Read the model definition and answer for the solid it produces. Units are mm, in the model's axes. A direction names the side the tool comes from. Give positions to 0.01 mm unless a question says otherwise; leave off trailing zeros. Order: outer loops, then holes, each group sorted by start corner. A loop starts at its lowest first (then second) coordinate and runs counter-clockwise, first axis right, second up. Notation, with made-up numbers: (39.25, 76.25) - (48.25, 76.25) arc R30 cw to (48.25, 106.25) - close; hole circle Ø3 at (67.25, -0.5). An arc over 180 degrees is marked (long way). Write item = value, one per line.
```python
from build123d import *

# Parameters (mm, degrees)
BOSS_EXTRU_1_DEPTH      = 4
ESQUISSE4_R             = 2.43
ENL_V_MAT_EXTRU_1_DEPTH = 2.7
ESQUISSE5_R             = 0.75
ENL_V_MAT_EXTRU_2_DEPTH = 1.3
CONG_1_R                = 1
ESQUISSE6_W             = 5.35
ESQUISSE6_H             = 23
BOSS_EXTRU_2_DEPTH      = 4
CONG_4_R                = 5.45
ENL_V_START             = -4
ENL_V_MAT_EXTRU_3_DEPTH = 4
CONG_5_R                = 2
CONG_6_R                = 2
CONG_7_R                = 1


with BuildPart() as part:
    # Esquisse3 → Boss.-Extru.1 (new body)
    with BuildSketch(Plane.XY):
        with BuildLine():
            Line((0, 0), (0, 65))
            Line((0, 65), (11.3, 65))
            Line((11.3, 65), (11.3, 11.3))
            Line((11.3, 11.3), (22.73, 11.3))
            Line((22.73, 11.3), (22.73, -23))
            ThreePointArc((22.73, -23), (17.08, -28.65), (11.43, -23))
            Line((11.43, -23), (11.43, 0))
            Line((11.43, 0), (0, 0))
        make_face()
    extrude(amount=BOSS_EXTRU_1_DEPTH)

    # Esquisse4 → Enlèv. mat.-Extru.1 (cut)
    with BuildSketch(Plane.XY.offset(4)):
        with Locations((17.08, -23)):
            Circle(ESQUISSE4_R)
    extrude(amount=-ENL_V_MAT_EXTRU_1_DEPTH, mode=Mode.SUBTRACT)

    # Esquisse5 → Enlèv. mat.-Extru.2 (cut)
    with BuildSketch(Plane.XY.offset(1.3)):
        with Locations((17.08, -23)):
            Circle(ESQUISSE5_R)
    extrude(amount=-ENL_V_MAT_EXTRU_2_DEPTH, mode=Mode.SUBTRACT)

    # Congé1
    cong_1_edges = [part.edges().sort_by_distance(p)[0] for p in [
        (0, 65, 2),
        (11.3, 65, 2),
    ]]
    fillet(cong_1_edges, radius=CONG_1_R)

    # Esquisse6 → Boss.-Extru.2 (add)
    with BuildSketch(Plane.XY.offset(4)):
        with Locations((8.755, -11.5)):
            Rectangle(ESQUISSE6_W, ESQUISSE6_H)
    extrude(amount=-BOSS_EXTRU_2_DEPTH)

    # Congé4
    # the kernel refuses this fillet: 5.45 mm, written as the material it takes off along each edge
    with BuildSketch(Plane(origin=(6.08, -23, 17.625), x_dir=(0, 1, 0), z_dir=(0, 0, -1))) as cong_4_piece_1_section:
        with BuildLine():
            CenterArc((CONG_4_R, CONG_4_R), CONG_4_R, 180, 90)
            Line((0, CONG_4_R), (0, 0))
            Line((0, 0), (CONG_4_R, 0))
        make_face()
    cong_4_piece_1 = extrude(amount=31.25, mode=Mode.PRIVATE)
    cong_4_piece_1 = cong_4_piece_1 - Plane(origin=(17.08, -23, 2), x_dir=(1, 0, 0), z_dir=(0, 0, -1)) * Cylinder(5.65, 85, mode=Mode.PRIVATE)
    add(cong_4_piece_1, mode=Mode.SUBTRACT)

    # Esquisse7 → Enlèv. mat.-Extru.3 (cut)
    with BuildSketch(Plane.XY.offset(4).offset(ENL_V_START)):
        with BuildLine():
            Line((17.08, -17.35), (17.08, 11.3))
            Line((17.08, 11.3), (22.73, 11.3))
            Line((22.73, 11.3), (22.73, -23))
            ThreePointArc((22.73, -23), (21.075153314, -19.004846686), (17.08, -17.35))
        make_face()
    extrude(amount=ENL_V_MAT_EXTRU_3_DEPTH, mode=Mode.SUBTRACT)

    # Congé5
    cong_5_edges = [part.edges().sort_by_distance(p)[0] for p in [
        (0, 0, 2),
        (17.08, 11.3, 2),
    ]]
    fillet(cong_5_edges, radius=CONG_5_R)

    # Congé6
    cong_6_edges = [part.edges().sort_by_distance(p)[0] for p in [
        (11.430000074, -22.999082493, 2),
        (17.08, -17.35, 2),
    ]]
    fillet(cong_6_edges, radius=CONG_6_R)

    # Congé7
    cong_7_edges = [part.edges().sort_by_distance(p)[0] for p in [
        (11.3, 37.65, 4),
        (0, 33, 0),
        (0, 33, 4),
        (5.65, 65, 0),
        (11.007106781, 64.707106781, 0),
        (0.292893219, 64.707106781, 0),
        (5.65, 65, 4),
        (11.007106781, 64.707106781, 4),
        (0.292893219, 64.707106781, 4),
        (6.08, -8.775, 0),
        (6.08, -8.775, 4),
        (7.213643754, -20.877396694, 4),
        (17.08, -3.158032367, 4),
        (17.08, -3.158032367, 0),
        (13.19, 11.3, 4),
        (4.04, 0, 4),
        (0.585786438, 0.585786438, 4),
        (16.494213562, 10.714213562, 4),
        (13.19, 11.3, 0),
        (4.04, 0, 0),
        (0.585786438, 0.585786438, 0),
        (16.494213562, 10.714213562, 0),
        (21.008529301, -27.060684367, 0),
        (11.3, 37.65, 0),
        (21.008529301, -27.060684367, 4),
        (7.213643754, -20.877396694, 0),
        (11.066365829, -23.35890716, 0),
        (11.066365829, -23.35890716, 4),
        (17.491643674, -16.831434713, 4),
        (17.491643674, -16.831434713, 0),
    ]]
    fillet(cong_7_edges, radius=CONG_7_R)


solid = part.part
```
1. Section A-A (y = 34) is taken. Determine the outline of the cut face in (x, z), and give its area (3 significant figures).
Recorded:
outline = (0, 1) arc R1 ccw to (1, 0) - (10.3, 0) arc R1 ccw to (11.3, 1) - (11.3, 3) arc R1 ccw to (10.3, 4) - (1, 4) arc R1 ccw to (0, 3) - close
area = 44.3 mm^2
2. For faces 1 (the face through (18.201, -25.156, 2.669)), 2 (the face through (9, 19, 4)), 3 (the face through (13, 11.3, 2)), 4 (the face through (6.08, -9, 2)), 5 (the face through (9, 19, 0)), determine the directions among +Z, -Z, +X, -X, +Y, -Y from which every point of the face is accessible in a straight line to the end or side of a thin tool.
Recorded:
face_1 = +Z
face_2 = +Z, +X, -X, +Y, -Y
face_3 = +Z, -Z, +X, +Y
face_4 = +Z, -Z, -X, -Y
face_5 = -Z, +X, -X, +Y, -Y
3. Determine the mould class of faces 6 (the face through (17.426, -23.665, 0.659)), 7 (the face through (4, 0, 2)), 8 (the face through (0, 33, 2)) for opening direction X: +X half, -X half, draft (parallel to the pull), parting line (faces both ways), or undercut.
Recorded:
face_6 = undercut
face_7 = draft
face_8 = -X half
4. Flat-ended cylindrical pins translate along their axes: pin 1 (2 mm diameter, centred on x = 12.5, z = 2.5, fed in from +Y); pin 2 (1 mm diameter, centred on x = 14.5, z = 0.5, fed in from -Y); pin 3 (2 mm diameter, centred on y = 49, z = 2, fed in from +X); pin 4 (0.9 mm diameter, centred on x = 17.08, y = -23, fed in from +Z). Find the tip coordinate at first contact, or state that the pin passes through.
Recorded:
pin_1 = 11.3
pin_2 = -28.19
pin_3 = 11.3
pin_4 = through
5. Straight lines are drawn through the part: L1, parallel to X at y = -5, z = 3; L2, parallel to Y at x = 7, z = 2.2; L3, parallel to X at y = 53, z = 1.3. For each, find the intervals that lie inside material, in ascending order. Write a range as [from, to].
Recorded:
L1 = [6.08, 17.08]
L2 = [-20.58, 65]
L3 = [0, 11.3]
6. Section B-B (y = 3) is taken. Determine the outline of the cut face in (x, z), and give its area (3 significant figures).
Recorded:
outline = (0, 1) arc R1 ccw to (1, 0) - (16.08, 0) arc R1 ccw to (17.08, 1) - (17.08, 3) arc R1 ccw to (16.08, 4) - (1, 4) arc R1 ccw to (0, 3) - close
area = 67.5 mm^2
